```python
from build123d import *

# Parameters (mm, degrees)
SKETCH1_W           = 88.9
SKETCH1_H           = 71.12
BOSS_EXTRUDE1_DEPTH = 60.96
SKETCH2_W           = 85.344
SKETCH2_H           = 67.564
CUT_EXTRUDE1_DEPTH  = 59.182
SKETCH3_R           = 2.286
CUT_EXTRUDE2_DEPTH  = 5.08
SKETCH4_R           = 2.794
BOSS_EXTRUDE2_DEPTH = 6.1214
SKETCH5_R           = 1.27
CUT_EXTRUDE3_DEPTH  = 3.81
SKETCH7_W           = 72.39
SKETCH7_H           = 25.3492
CUT_EXTRUDE5_DEPTH  = 4.699
SKETCH8_R           = 3.175
BOSS_EXTRUDE3_DEPTH = 7.999555
SKETCH9_R           = 1.27
CUT_EXTRUDE6_DEPTH  = 3.81
SKETCH11_R          = 2.032
SKETCH11_R_2        = 5.08
CUT_EXTRUDE7_DEPTH  = 5.08
SKETCH12_R          = 3.81
CUT_EXTRUDE8_DEPTH  = 3.302
BOSS_EXTRUDE4_DEPTH = 59.182
SKETCH14_R          = 1.27
CUT_EXTRUDE9_DEPTH  = 3.81


with BuildPart() as part:
    # Sketch1 → Boss-Extrude1 (new body)
    with BuildSketch(Plane.XY):
        Rectangle(SKETCH1_W, SKETCH1_H)
    extrude(amount=BOSS_EXTRUDE1_DEPTH)

    # Sketch2 → Cut-Extrude1 (cut)
    with BuildSketch(Plane(origin=(0, 0, 0), x_dir=(-1, 0, 0), z_dir=(0, 0, -1))):
        Rectangle(SKETCH2_W, SKETCH2_H)
    extrude(amount=-CUT_EXTRUDE1_DEPTH, mode=Mode.SUBTRACT)

    # Sketch3 → Cut-Extrude2 (cut)
    with BuildSketch(Plane.XY.offset(60.96)):
        with Locations((-18.0975, -7.4676)):
            Circle(SKETCH3_R)
        with Locations((-5.9055, -7.4676)):
            Circle(SKETCH3_R)
        with Locations((5.9055, -7.4676)):
            Circle(SKETCH3_R)
        with Locations((18.0975, -7.4676)):
            Circle(SKETCH3_R)
    extrude(amount=-CUT_EXTRUDE2_DEPTH, mode=Mode.SUBTRACT)

    # Sketch4 → Boss-Extrude2 (add)
    with BuildSketch(Plane(origin=(0, 0, 59.182), x_dir=(-1, 0, 0), z_dir=(0, 0, -1))):
        with Locations((-23.1013, -1.778)):
            Circle(SKETCH4_R)
        with Locations((23.1013, -1.778)):
            Circle(SKETCH4_R)
        with Locations((23.1013, -30.0228)):
            Circle(SKETCH4_R)
        with Locations((-23.1013, -30.0228)):
            Circle(SKETCH4_R)
    extrude(amount=BOSS_EXTRUDE2_DEPTH)

    # Sketch5 → Cut-Extrude3 (cut)
    with BuildSketch(Plane(origin=(0, 0, 53.0606), x_dir=(-1, 0, 0), z_dir=(0, 0, -1))):
        with Locations((-23.1013, -1.778)):
            Circle(SKETCH5_R)
        with Locations((23.1013, -1.778)):
            Circle(SKETCH5_R)
        with Locations((23.1013, -30.0228)):
            Circle(SKETCH5_R)
        with Locations((-23.1013, -30.0228)):
            Circle(SKETCH5_R)
    extrude(amount=-CUT_EXTRUDE3_DEPTH, mode=Mode.SUBTRACT)

    # Sketch7 → Cut-Extrude5 (cut)
    with BuildSketch(Plane.XY.offset(60.96)):
        with Locations((0, 14.862768706)):
            Rectangle(SKETCH7_W, SKETCH7_H)
    extrude(amount=-CUT_EXTRUDE5_DEPTH, mode=Mode.SUBTRACT)

    # Sketch8 → Boss-Extrude3 (add)
    with BuildSketch(Plane(origin=(0, 0, 59.182), x_dir=(-1, 0, 0), z_dir=(0, 0, -1))):
        with Locations((-37.5285, 30.5435)):
            Circle(SKETCH8_R)
        with Locations((37.5285, 30.5435)):
            Circle(SKETCH8_R)
        with Locations((37.5285, -0.6985)):
            Circle(SKETCH8_R)
        with Locations((-37.5285, -0.6985)):
            Circle(SKETCH8_R)
    extrude(amount=BOSS_EXTRUDE3_DEPTH)

    # Sketch9 → Cut-Extrude6 (cut)
    with BuildSketch(Plane(origin=(0, 0, 51.182445152), x_dir=(-1, 0, 0), z_dir=(0, 0, -1))):
        with Locations((-37.5285, 30.5435)):
            Circle(SKETCH9_R)
        with Locations((37.5285, 30.5435)):
            Circle(SKETCH9_R)
        with Locations((37.5285, -0.6985)):
            Circle(SKETCH9_R)
        with Locations((-37.5285, -0.6985)):
            Circle(SKETCH9_R)
    extrude(amount=-CUT_EXTRUDE6_DEPTH, mode=Mode.SUBTRACT)

    # Sketch11 → Cut-Extrude7 (cut)
    with BuildSketch(Plane(origin=(0, 35.56, 0), x_dir=(1, 0, 0), z_dir=(0, 1, 0))):
        with Locations(Location((-6.732036627, -12.594763228, 0), (0, 0, 270))):
            Circle(SKETCH11_R)
        with Locations(Location((17.765022524, -37.523151726, 0), (0, 0, 270))):
            Circle(SKETCH11_R)
        with Locations(Location((0, -30.48, 0), (0, 0, 270))):
            Circle(SKETCH11_R_2)
    extrude(amount=-CUT_EXTRUDE7_DEPTH, mode=Mode.SUBTRACT)

    # Sketch12 → Cut-Extrude8 (cut)
    with BuildSketch(Plane.ZY.offset(44.45)):
        with Locations((10.16, -22.86)):
            Circle(SKETCH12_R)
    extrude(amount=-CUT_EXTRUDE8_DEPTH, mode=Mode.SUBTRACT)

    # Sketch13 → Boss-Extrude4 (add)
    with BuildSketch(Plane(origin=(0, 0, 59.182), x_dir=(-1, 0, 0), z_dir=(0, 0, -1))):
        with BuildLine():
            Line((42.672, 25.346634714), (42.672, 19.209934994))
            ThreePointArc((42.672, 19.209934994), (40.312998858, 22.278284854), (42.672, 25.346634714))
        make_face()
        with BuildLine():
            Line((44.45, -29.023311525), (44.45, -35.56))
            Line((44.45, -35.56), (37.913311525, -35.56))
            ThreePointArc((37.913311525, -35.56), (39.079897552, -30.189897552), (44.45, -29.023311525))
        make_face()
        with BuildLine():
            Line((-42.672, 25.346634714), (-42.672, 19.209934994))
            ThreePointArc((-42.672, 19.209934994), (-40.312998858, 22.278284854), (-42.672, 25.346634714))
        make_face()
        with BuildLine():
            Line((-44.45, -29.023311525), (-44.45, -35.56))
            Line((-44.45, -35.56), (-37.913311525, -35.56))
            ThreePointArc((-37.913311525, -35.56), (-39.079897552, -30.189897552), (-44.45, -29.023311525))
        make_face()
    extrude(amount=BOSS_EXTRUDE4_DEPTH)

    # Sketch14 → Cut-Extrude9 (cut)
    with BuildSketch(Plane(origin=(0, 0, 0), x_dir=(-1, 0, 0), z_dir=(0, 0, -1))):
        with Locations((-42.344998858, 22.278284854)):
            Circle(SKETCH14_R)
        with Locations((-41.275, -32.385)):
            Circle(SKETCH14_R)
        with Locations((41.275, -32.385)):
            Circle(SKETCH14_R)
        with Locations((42.344998858, 22.278284854)):
            Circle(SKETCH14_R)
    extrude(amount=-CUT_EXTRUDE9_DEPTH, mode=Mode.SUBTRACT)


solid = part.part
```
Geometry check sheet. Reference: the model listing, model coordinates, mm. A direction names the side the tool comes from. Coordinates: 2 decimals unless noted, no trailing zeros. Order: outer loops, then holes, each group sorted by start corner. A loop starts at its lowest first (then second) coordinate and runs counter-clockwise, first axis right, second up. Notation, with made-up numbers: (32, 29) - (38, 29) arc R29 ccw to (38, 55) - close; hole circle Ø7 at (7.5, 84). An arc over 180 degrees is marked (long way). Answer as a JSON object with one key per item and string values. Group by question number.
Item 1: Scan lines: probe 1 along X at (y, z) = (-12, 41); probe 2 along Y at (x, z) = (-5, 23). Record each from-to range of solid material in increasing order.
Item 2: Sectioned sample at A-A, the plane x = 13. Record the cut outline in (y, z), and give its area (3 significant figures).
Item 3: Sectioned sample at B-B, the plane y = -22.86. Record the cut outline in (x, z), and give its area (3 significant figures).
Item 4: Draft check along X on faces 1 (the face through (44.45, 0, 30)), 2 (the face through (-24, -3, 53.061)), 3 (the face through (-44.45, 0, 30)). Enter one of: +X half, -X half, draft (parallel to the pull), parting line (faces both ways), or undercut.
Item 5: Depth check by flat-ended pin: pin 1 Ø1.9 at (x, y) = (-37.5, -1.5) entering from -Z; pin 2 Ø3.5 at (x, y) = (42.34, 22.28) entering from -Z; pin 3 Ø10 at (x, y) = (-5.5, -26) entering from -Z; pin 4 Ø1.3 at (x, y) = (-42, 22) entering from -Z. Enter the tip coordinate at first touch or a pass-through.
Item 6: Sectioned sample at D-D, the plane y = -11. Record the cut outline in (x, z), and give its area (3 significant figures).
Item 7: Sectioned sample at C-C, the plane x = 0. Record the cut outline in (y, z), and give its area (3 significant figures).
Item 8: Tool access check on faces 4 (the face through (15.814, -7.367, 60.083)), 5 (the face through (-7.51, 34.68, 14.47)), 6 (the face through (42.62, 21.04, 1.88)). Record the directions out of +Z, -Z, +X, -X, +Y, -Y that give a thin tool (end or side, any length) a straight path to the whole face; none if there is none.
Resolved:
{
 "1": {"probe 1": "-44.45 to -42.67, 42.67 to 44.45", "probe 2": "-35.56 to -33.78, 33.78 to 35.56"},
 "2": {"outline": "(-35.56, 0) - (-33.78, 0) - (-33.78, 59.18) - (2.19, 59.18) - (2.19, 60.96) - (-35.56, 60.96) - close; (27.54, 59.18) - (33.78, 59.18) - (33.78, 0) - (35.56, 0) - (35.56, 60.96) - (27.54, 60.96) - close", "area": "292 mm^2"},
 "3": {"outline": "(-44.45, 0) - (-42.67, 0) - (-42.67, 6.35) - (-44.45, 6.35) - close; (-44.45, 13.97) - (-42.67, 13.97) - (-42.67, 59.18) - (42.67, 59.18) - (42.67, 0) - (44.45, 0) - (44.45, 60.96) - (-44.45, 60.96) - close", "area": "355 mm^2"},
 "4": {"face 1": "+X half", "face 2": "undercut", "face 3": "-X half"},
 "5": {"pin 1": "z = 51.18", "pin 2": "z = 0", "pin 3": "z = 59.18", "pin 4": "z = 3.81"},
 "6": {"outline": "(-44.45, 0) - (-42.67, 0) - (-42.67, 59.18) - (42.67, 59.18) - (42.67, 0) - (44.45, 0) - (44.45, 60.96) - (-44.45, 60.96) - close", "area": "369 mm^2"},
 "7": {"outline": "(-35.56, 0) - (-33.78, 0) - (-33.78, 59.18) - (2.19, 59.18) - (2.19, 60.96) - (-35.56, 60.96) - close; (27.54, 59.18) - (33.78, 59.18) - (33.78, 35.56) - (35.56, 35.56) - (35.56, 60.96) - (27.54, 60.96) - close; (33.78, 0) - (35.56, 0) - (35.56, 25.4) - (33.78, 25.4) - close", "area": "274 mm^2"},
 "8": {"face 4": "+Z, -Z", "face 5": "+Y", "face 6": "-Z"}
}
